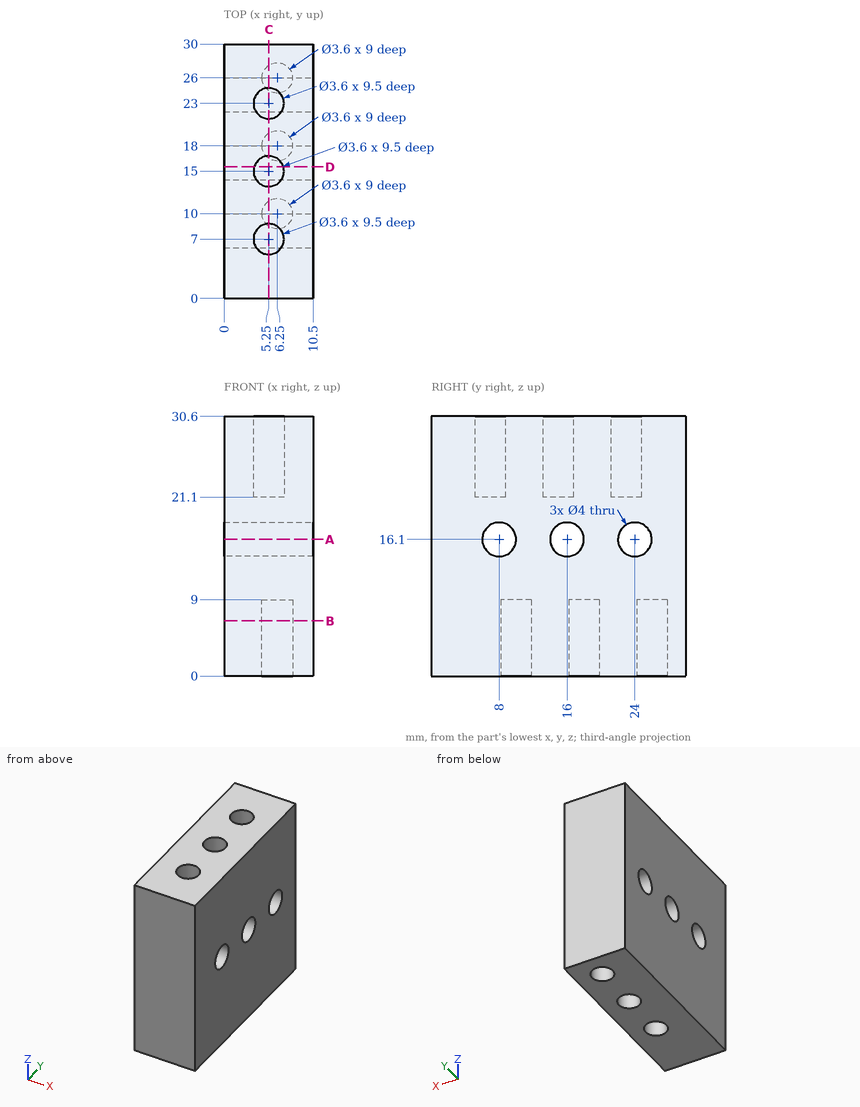
Input: dimensioned drawing with shaded views. Units: mm. Origin: part minimum x, y, z. Round coordinates to 2 decimals unless told otherwise and drop trailing zeros. Loops run counter-clockwise (first coordinate to the right, second up) from the corner with the lowest first, then second, coordinate; pieces in that order, holes last. Notation, with made-up numbers: (-22, 16) -> (13, 16) arc R22 ccw to (13, 25) -> close; hole circle Ø5 at (14, 49). An arc over 180 degrees is marked (long way). One line per item, written item: value.
(1) Section C-C (x = 5.25). Give the number of separate pieces and of enclosed holes in the cut face, plus the area to 3 significant figures.
Geometry check:
separate pieces: 1
enclosed holes: 3
area: 697 mm2
(2) Material intervals for line 1 (Y direction, x = 6.25, z = 4.5); line 2 (Y direction, x = 5.25, z = 23.75); line 3 (Z direction, x = 6.5, y = 19.25), sorted ascending. Write a range as [from, to].
Geometry check:
line 1: [0, 8.2], [11.8, 16.2], [19.8, 24.2], [27.8, 30]
line 2: [0, 5.2], [8.8, 13.2], [16.8, 21.2], [24.8, 30]
line 3: [9, 30.6]
(3) Pin query (flat end, axial travel): pin 1 (3 mm diameter, centred on x = 6.25, y = 26, fed in from -Z); pin 2 (1.8 mm diameter, centred on x = 4.5, y = 7, fed in from +Z); pin 3 (3.5 mm diameter, centred on y = 16, z = 16.1, fed in from +X). Return the tip coordinate at first contact, or that it passes through.
Geometry check:
pin 1: z = 9
pin 2: z = 21.1
pin 3: through
(4) Section A-A (z = 16.1). Return the cut outline in (x, y).
Geometry check:
outline: (0, 0) -> (10.5, 0) -> (10.5, 6) -> (0, 6) -> close; (0, 10) -> (10.5, 10) -> (10.5, 14) -> (0, 14) -> close; (0, 18) -> (10.5, 18) -> (10.5, 22) -> (0, 22) -> close; (0, 26) -> (10.5, 26) -> (10.5, 30) -> (0, 30) -> close
(5) Section B-B (z = 6.5). Return the cut outline in (x, y).
Geometry check:
outline: (0, 0) -> (10.5, 0) -> (10.5, 30) -> (0, 30) -> close; hole circle Ø3.6 at (6.25, 10); hole circle Ø3.6 at (6.25, 18); hole circle Ø3.6 at (6.25, 26)
(6) Section D-D (y = 15.5). Return the cut outline in (x, z), plus the area to 3 significant figures.
Geometry check:
outline: (0, 0) -> (10.5, 0) -> (10.5, 14.16) -> (0, 14.16) -> close; (0, 18.04) -> (10.5, 18.04) -> (10.5, 30.6) -> (6.98, 30.6) -> (6.98, 21.1) -> (3.52, 21.1) -> (3.52, 30.6) -> (0, 30.6) -> close
area: 248 mm2
